The model under review builds one solid part; all positions refer to its coordinate system, in mm. A direction names the side the tool comes from. Coordinates: 2 decimals unless noted, no trailing zeros. Order: outer loops, then holes, each group sorted by start corner. A loop starts at its lowest first (then second) coordinate and runs counter-clockwise, first axis right, second up.
```python
from build123d import *

# Parameters (mm, degrees)
SKETCH1_W           = 76.2
SKETCH1_H           = 114.3
BOSS_EXTRUDE1_DEPTH = 3.175
SKETCH3_W           = 76.2
SKETCH3_H           = 114.3
SKETCH3_W_2         = 63.5
SKETCH3_H_2         = 101.6
BOSS_EXTRUDE2_DEPTH = 25.4
CUT_EXTRUDE1_REACH  = 116.3
SKETCH4_R           = 3.175
SKETCH4_W           = 11.43
SKETCH4_H           = 8.89
SKETCH5_W           = 68.58
SKETCH5_H           = 106.68
SKETCH5_W_2         = 63.5
SKETCH5_H_2         = 101.6
BOSS_EXTRUDE3_DEPTH = 6.35
FILLET3_R           = 6.35
FILLET4_R           = 4.7625
FILLET5_R           = 3.175
FILLET6_R           = 0.79375
SKETCH6_R           = 4.7625
BOSS_EXTRUDE4_DEPTH = 31.75
SKETCH8_R           = 1.4986
CUT_EXTRUDE2_DEPTH  = 12.7
FILLET8_R           = 2.54


with BuildPart() as part:
    # Sketch1 → Boss-Extrude1 (new body)
    with BuildSketch(Plane(origin=(0, 0, 0), x_dir=(1, 0, 0), z_dir=(0, 1, 0))):
        Rectangle(SKETCH1_W, SKETCH1_H)
    extrude(amount=BOSS_EXTRUDE1_DEPTH)

    # Sketch3 → Boss-Extrude2 (add)
    with BuildSketch(Plane(origin=(0, 3.175, 0), x_dir=(1, 0, 0), z_dir=(0, 1, 0))):
        Rectangle(SKETCH3_W, SKETCH3_H)
        Rectangle(SKETCH3_W_2, SKETCH3_H_2, mode=Mode.SUBTRACT)
    extrude(amount=BOSS_EXTRUDE2_DEPTH)

    # Sketch4 → Cut-Extrude1 (cut, up to next)
    with BuildSketch(Plane.XY.offset(57.15), mode=Mode.PRIVATE) as cut_extrude1_sk1:
        with Locations((-18.288, 18.415)):
            Circle(SKETCH4_R)
    cut_extrude1_tool1 = extrude(cut_extrude1_sk1.sketch, amount=-CUT_EXTRUDE1_REACH, mode=Mode.PRIVATE) & part.part
    add(cut_extrude1_tool1.solids().sort_by_distance((-18.288, 18.415, 57.15))[0], mode=Mode.SUBTRACT)
    # Sketch4 → Cut-Extrude1 (cut, up to next)
    with BuildSketch(Plane.XY.offset(57.15), mode=Mode.PRIVATE) as cut_extrude1_sk2:
        with Locations((-5.588, 18.415)):
            Rectangle(SKETCH4_W, SKETCH4_H)
    cut_extrude1_tool2 = extrude(cut_extrude1_sk2.sketch, amount=-CUT_EXTRUDE1_REACH, mode=Mode.PRIVATE) & part.part
    add(cut_extrude1_tool2.solids().sort_by_distance((-5.588, 18.415, 57.15))[0], mode=Mode.SUBTRACT)

    # Sketch5 → Boss-Extrude3 (add)
    with BuildSketch(Plane(origin=(0, 28.575, 0), x_dir=(1, 0, 0), z_dir=(0, 1, 0))):
        Rectangle(SKETCH5_W, SKETCH5_H)
        Rectangle(SKETCH5_W_2, SKETCH5_H_2, mode=Mode.SUBTRACT)
    extrude(amount=BOSS_EXTRUDE3_DEPTH)

    # Fillet3
    fillet3_edges = [part.edges().sort_by_distance(p)[0] for p in [
        (38.1, 14.2875, 57.15),
        (-38.1, 14.2875, 57.15),
        (-38.1, 14.2875, -57.15),
        (38.1, 14.2875, -57.15),
    ]]
    fillet(fillet3_edges, radius=FILLET3_R)

    # Fillet4
    fillet4_edges = [part.edges().sort_by_distance(p)[0] for p in [
        (-34.29, 31.75, -53.34),
        (-34.29, 31.75, 53.34),
        (34.29, 31.75, 53.34),
        (34.29, 31.75, -53.34),
    ]]
    fillet(fillet4_edges, radius=FILLET4_R)

    # Fillet5
    fillet5_edges = [part.edges().sort_by_distance(p)[0] for p in [
        (-31.75, 19.05, 50.8),
        (31.75, 19.05, 50.8),
        (31.75, 19.05, -50.8),
        (-31.75, 19.05, -50.8),
    ]]
    fillet(fillet5_edges, radius=FILLET5_R)

    # Fillet6
    fillet6_edges = [part.edges().sort_by_distance(p)[0] for p in [
        (0.127, 22.86, 53.975),
        (0.127, 13.97, 53.975),
        (-11.303, 13.97, 53.975),
        (-11.303, 22.86, 53.975),
    ]]
    fillet(fillet6_edges, radius=FILLET6_R)

    # Sketch6 → Boss-Extrude4 (add)
    with BuildSketch(Plane(origin=(0, 3.175, 0), x_dir=(1, 0, 0), z_dir=(0, 1, 0))):
        with Locations((-29.5275, 48.5775)):
            Circle(SKETCH6_R)
        with Locations((29.5275, 48.5775)):
            Circle(SKETCH6_R)
        with Locations((29.5275, -48.5775)):
            Circle(SKETCH6_R)
        with Locations((-29.5275, -48.5775)):
            Circle(SKETCH6_R)
    extrude(amount=BOSS_EXTRUDE4_DEPTH)

    # Sketch8 → Cut-Extrude2 (cut)
    with BuildSketch(Plane(origin=(0, 34.925, 0), x_dir=(1, 0, 0), z_dir=(0, 1, 0))):
        with Locations((-29.5275, 48.5775)):
            Circle(SKETCH8_R)
        with Locations((29.5275, 48.5775)):
            Circle(SKETCH8_R)
        with Locations((29.5275, -48.5775)):
            Circle(SKETCH8_R)
        with Locations((-29.5275, -48.5775)):
            Circle(SKETCH8_R)
    extrude(amount=-CUT_EXTRUDE2_DEPTH, mode=Mode.SUBTRACT)

    # Fillet8
    fillet8_edges = [part.edges().sort_by_distance(p)[0] for p in [
        (-31.75, 19.05, -44.365386516),
        (-25.315386516, 19.05, -50.8),
        (25.315386516, 19.05, -50.8),
        (31.75, 19.05, -44.365386516),
        (31.75, 19.05, 44.365386516),
        (25.315386516, 19.05, 50.8),
        (-25.315386516, 19.05, 50.8),
        (-31.75, 19.05, 44.365386516),
    ]]
    fillet(fillet8_edges, radius=FILLET8_R)


solid = part.part
```
(1) Wall thickness on probe 1 along X at (y, z) = (27, 19.5); probe 2 along Z at (x, y) = (-11.5, 31.5); probe 3 along Z at (x, y) = (-20, 5): over which ranges is each line inside the solid? List them lowest first.
A:
probe 1: x = -38.1 to -31.75, 31.75 to 38.1
probe 2: z = -53.34 to -50.8, 50.8 to 53.34
probe 3: z = -57.15 to -50.8, 50.8 to 57.15
(2) We need section D-D, the plane y = 25.5. Count the separate pieces of the cut face and the enclosed holes in it, and give its area (3 significant figures).
A:
separate pieces: 1
enclosed holes: 5
area: 2,380 mm2
(3) Draft analysis for pull direction Z (two halves, no side actions). For faces 4 (the face through (-11.303, 18, 54)), 5 (the face through (-31.06, 18.83, 43.02)), 6 (the face through (0, 14, -57.15)), state which applies: released by +Z, released by -Z, zero draft, split by the parting line, or undercut.
A:
face 4: zero draft
face 5: undercut
face 6: released by -Z
(4) We need section C-C, the plane x = -13.5. Write out the cut boundary in (y, z) (3 decimals), and give its area (3 significant figures).
A:
outline: (0, -57.15) - (28.575, -57.15) - (28.575, -53.34) - (34.925, -53.34) - (34.925, -50.8) - (3.175, -50.8) - (3.175, 50.8) - (34.925, 50.8) - (34.925, 53.34) - (28.575, 53.34) - (28.575, 57.15) - (0, 57.15) - close
area: 718 mm2
(5) We need section B-B, the plane z = 2.5. Write out the cut boundary in (x, y) (3 decimals), and give its area (3 significant figures).
A:
outline: (-38.1, 0) - (38.1, 0) - (38.1, 28.575) - (34.29, 28.575) - (34.29, 34.925) - (31.75, 34.925) - (31.75, 3.175) - (-31.75, 3.175) - (-31.75, 34.925) - (-34.29, 34.925) - (-34.29, 28.575) - (-38.1, 28.575) - close
area: 597 mm2
(6) Machinability: for faces 1 (the face through (31.06, 18.83, -43.02)), 2 (the face through (-34.29, 32, 1)), 3 (the face through (32.86, 31.79, 51.98)), which of the approach directions +Z, -Z, +X, -X, +Y, -Y give a long, thin tool a straight path to every point of the face, cutting with its end or side? Answer none if there is none.
A:
face 1: +Y
face 2: +Z, -Z, -X, +Y
face 3: +Z, +X, +Y
(7) For pin 1 Ø1.5 at (x, z) = (29.5, -48) entering from +Y (3 decimals); pin 2 Ø4 at (x, z) = (8, 24.5) entering from +Y (3 decimals); pin 3 Ø1.9 at (x, y) = (-7.5, 31) entering from +Z, all flat-tipped, find the tip position at first contact; note any pin that passes through.
A:
pin 1: stops at y = 22.225
pin 2: stops at y = 3.175
pin 3: stops at z = 53.34
